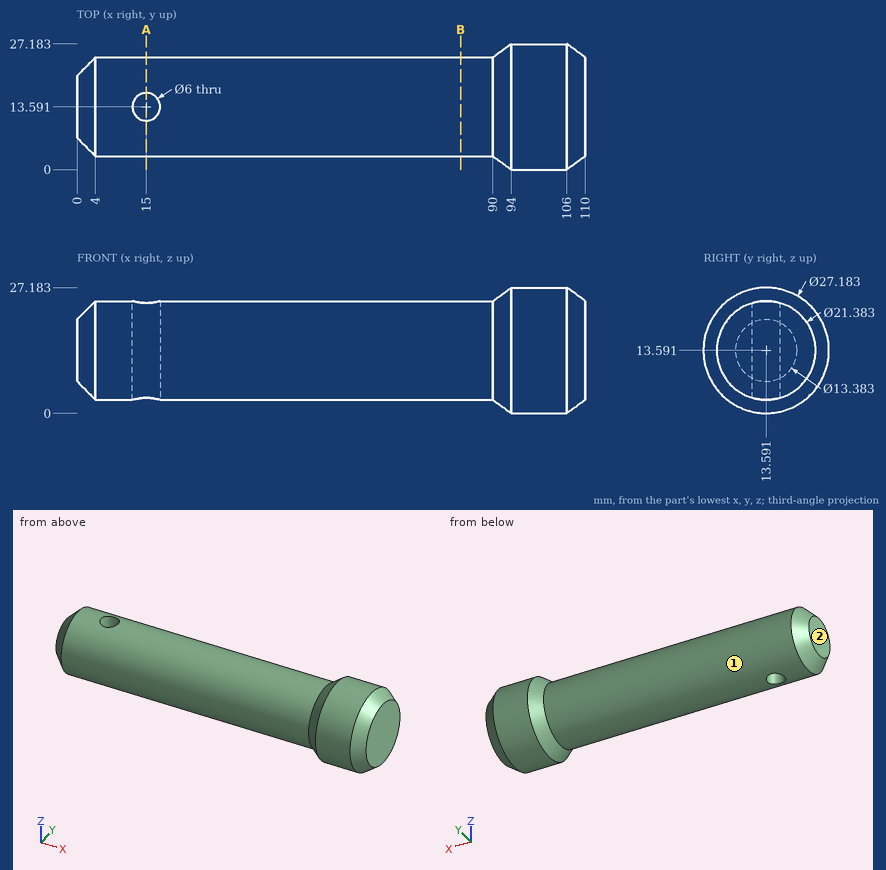
Check sheet for the drawn part. Datum: minimum x, y, z corner. Units: mm. A direction names the side the tool comes from. Give positions to 0.01 mm unless a question says otherwise; leave off trailing zeros. Order: outer loops, then holes, each group sorted by start corner. A loop starts at its lowest first (then second) coordinate and runs counter-clockwise, first axis right, second up.
1. Depth check by flat-ended pin: pin 1 (10 mm diameter, centred on x = 80, z = 17.5, fed in from +Y); pin 2 (8 mm diameter, centred on x = 15, y = 13.59, fed in from +Z); pin 3 (2 mm diameter, centred on x = 22.5, z = 17.5, fed in from +Y). Enter the tip coordinate at first touch or a pass-through.
Completed:
pin 1: stops at y = 24.28
pin 2: stops at z = 24.28
pin 3: stops at y = 23.88
2. Scan lines: line 1 (Y direction, x = 15, z = 18.75) (1 decimal); line 2 (Y direction, x = 75.5, z = 14) (1 decimal); line 3 (Y direction, x = 63.5, z = 12.5) (1 decimal). Record each from-to range of solid material in increasing order.
Completed:
line 1: y = 4.2 to 10.6, 16.6 to 23
line 2: y = 2.9 to 24.3
line 3: y = 3 to 24.2
3. Sectioned sample at B-B (x = 83). Record the boundary of the cut face in (y, z), then the cut area to 3 significant figures.
Completed:
outline: circle Ø21.38 at (13.59, 13.59)
area: 359 mm2
4. Access from +Z, -Z, +X, -X, +Y, -Y to the whole of each face (thin tool, end or side, straight path). Record for the marked faces 1 and 2.
Completed:
face 1: -X
face 2: +Z, -Z, -X, +Y, -Y
5. Sectioned sample at A-A (x = 15). Record the boundary of the cut face in (y, z).
Completed:
outline: (10.59, 3.33) - (10.59, 23.85) arc R10.69 ccw to start; (16.59, 3.33) arc R10.69 ccw to (16.59, 23.85) - close
